For this review, take the finished solid that the model builds, in its own axes (mm). Face numbers are marked on the shaded views. A direction names the side the tool comes from. Coordinates: 2 decimals unless noted, no trailing zeros. Loops run counter-clockwise (first coordinate to the right, second up) from the corner with the lowest first, then second, coordinate; pieces in that order, holes last. Notation, with made-up numbers: (75.25, 5) -> (104.25, 5) arc R12 ccw to (104.25, 17) -> close; hole circle Ø4 at (23.25, 35). An arc over 180 degrees is marked (long way). Answer in a Markdown table with one row per item.
from build123d import *

# Parameters (mm, degrees)
RESSALTO_EXTRUS_O1_DEPTH = 10
ESBO_O3_R                = 2
CORTE_EXTRUS_O1_DEPTH    = 15
CHANFRO1_SIZE            = 1.6
FILETE1_R                = 0.5
FILETE2_R                = 0.94
RESSALTO_EXTRUS_O3_DEPTH = 10
CHANFRO5_SIZE            = 2
CHANFRO4_SIZE            = 1


with BuildPart() as part:
    # Esboço1 → Ressalto-extrusão1 (new body)
    with BuildSketch(Plane.XY):
        with BuildLine():
            Line((57, 14.25), (1.2, 14.25))
            Line((1.2, 14.25), (1.2, 4.25))
            Line((1.2, 4.25), (7.2, 4.25))
            Line((7.2, 4.25), (7.2, -0.75))
            Line((7.2, -0.75), (1.2, -0.75))
            Line((1.2, -0.75), (1.2, -15.95))
            Line((1.2, -15.95), (21.2, -15.95))
            Line((21.2, -15.95), (21.2, -20.95))
            Line((21.2, -20.95), (-3.8, -20.95))
            Line((-3.8, -20.95), (-3.8, 19.25))
            Line((-3.8, 19.25), (52, 19.25))
            Line((52, 19.25), (52, 16.25))
            Line((52, 16.25), (56.504380809, 16.25))
            ThreePointArc((56.504380809, 16.25), (56.67525574, 16.362291088), (56.829148206, 16.496918869))
            ThreePointArc((56.829148206, 16.496918869), (56.938176044, 16.51877572), (57, 16.426349589))
            Line((57, 16.426349589), (57, 16.25))
            Line((57, 16.25), (57, 14.25))
        make_face()
    extrude(amount=RESSALTO_EXTRUS_O1_DEPTH)

    # Esboço3 → Corte-extrusão1 (cut)
    with BuildSketch(Plane.XZ.offset(20.95)):
        with Locations(Location((13.2, 5, 0), (0, 0, 270))):
            Circle(ESBO_O3_R)
    extrude(amount=-CORTE_EXTRUS_O1_DEPTH, mode=Mode.SUBTRACT)

    # Chanfro1
    chanfro1_edges = [part.edges().sort_by_distance(p)[0] for p in [
        (13.2, -20.95, 7),
    ]]
    chamfer(chanfro1_edges, length=CHANFRO1_SIZE)

    # Filete1
    filete1_edges = [part.edges().sort_by_distance(p)[0] for p in [
        (13.2, -15.95, 7),
    ]]
    fillet(filete1_edges, radius=FILETE1_R)

    # Filete2
    filete2_edges = [part.edges().sort_by_distance(p)[0] for p in [
        (52, 16.25, 5),
    ]]
    fillet(filete2_edges, radius=FILETE2_R)

    # Esboço5 → Ressalto-extrusão3 (add)
    with BuildSketch(Plane.XY.offset(10)):
        Polygon((52, 19.25), (52, 21.25), (50, 21.25), (48, 19.25), align=None)
    extrude(amount=-RESSALTO_EXTRUS_O3_DEPTH)

    # Chanfro5
    chanfro5_edges = [part.edges().sort_by_distance(p)[0] for p in [
        (21.2, -20.95, 5),
        (-3.8, -20.95, 5),
        (-3.8, 19.25, 5),
        (7.2, 4.25, 5),
    ]]
    chamfer(chanfro5_edges, length=CHANFRO5_SIZE)

    # Chanfro4
    chanfro4_edges = [part.edges().sort_by_distance(p)[0] for p in [
        (1.2, 9.25, 10),
        (29.1, 14.25, 10),
        (29.1, 14.25, 0),
        (1.2, 9.25, 0),
        (7.2, 0.75, 0),
        (57, 14.25, 5),
        (7.2, 0.75, 10),
        (23.1, 19.25, 0),
        (23.1, 19.25, 10),
        (49, 20.25, 10),
        (49, 20.25, 0),
        (8.7, -20.95, 0),
        (8.7, -20.95, 10),
        (21.2, -17.45, 0),
        (-3.8, -0.85, 0),
        (3.2, 4.25, 0),
        (-2.8, 18.25, 0),
        (6.2, 3.25, 0),
        (20.2, -19.95, 0),
        (-2.8, -19.95, 0),
        (-3.8, -0.85, 10),
        (3.2, 4.25, 10),
        (21.2, -17.45, 10),
        (-2.8, 18.25, 10),
        (6.2, 3.25, 10),
        (20.2, -19.95, 10),
        (-2.8, -19.95, 10),
    ]]
    chamfer(chanfro4_edges, length=CHANFRO4_SIZE)


solid = part.part
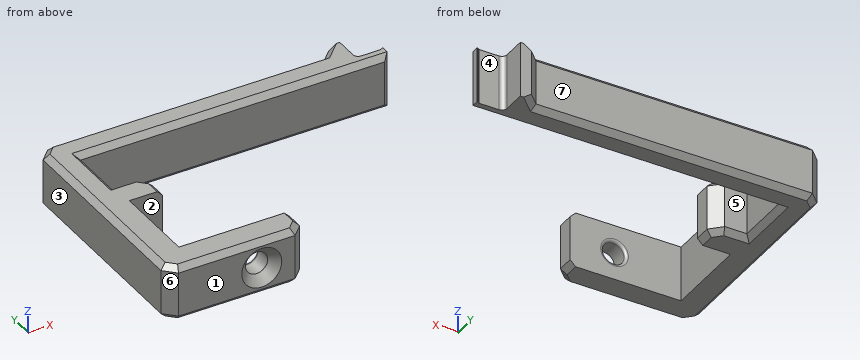
Item 1: Insertion check: pin 1 (5 mm diameter, centred on x = 14.5, z = 3.5, fed in from +Y); pin 2 (1.5 mm diameter, centred on y = -17.5, z = 3, fed in from +X); pin 3 (3 mm diameter, centred on y = -7.5, z = 4.5, fed in from +X). Each pin has a flat end and moves straight along its axis. Give the tip position at first contact, or say it passes through.
Worked answers:
| item | result |
|---|---|
| pin 1 | y = 19.25 |
| pin 2 | x = 21.2 |
| pin 3 | x = 1.2 |
Item 2: Take a section at D-D, the plane x = 44. State the section outline as (y, z) points.
Worked answers:
| item | result |
|---|---|
| outline | (14.25, 1) -> (15.25, 0) -> (18.25, 0) -> (19.25, 1) -> (19.25, 9) -> (18.25, 10) -> (15.25, 10) -> (14.25, 9) -> close |
Item 3: The part is to be moulded in two halves that separate along Y. For the marked faces 1, 2, 3 and 4, say which applies: +Y half, -Y half, draft (parallel to the pull), parting line (faces both ways), or undercut.
Worked answers:
| item | result |
|---|---|
| face 1 | -Y half |
| face 2 | undercut |
| face 3 | draft |
| face 4 | +Y half |
Item 4: For L1, parallel to Y at x = 6, z = 0.5; L2, parallel to Z at x = 13, y = -17; L3, parallel to Y at x = 9.5, z = 4, list the stretches that pass through material, from the lowest coordinate up.
Worked answers:
| item | result |
|---|---|
| L1 | -20.45 to -15.95, -0.75 to 2.74, 14.75 to 18.75 |
| L2 | 0 to 3.01, 6.99 to 10 |
| L3 | -20.95 to -15.95, 14.25 to 19.25 |
Item 5: For the marked faces 5, 6 and 7, list the 3-axis set-ups (+Z, -Z, +X, -X, +Y, -Y) from which the entire face can be reached by the end or side of a thin tool; tool diameter is ignored.
Worked answers:
| item | result |
|---|---|
| face 5 | +Z, -Z, +X |
| face 6 | +Z, -Z, -X, -Y |
| face 7 | +Z, -Z, -X, +Y |
Item 6: Take a section at C-C, the plane y = 12. State the section outline as (x, z) points.
Worked answers:
| item | result |
|---|---|
| outline | (-3.8, 1) -> (-2.8, 0) -> (0.2, 0) -> (1.2, 1) -> (1.2, 9) -> (0.2, 10) -> (-2.8, 10) -> (-3.8, 9) -> close |
Item 7: Take a section at A-A, the plane x = 13.2. State the section outline as (y, z) points, and give its area (3 significant figures).
Worked answers:
| item | result |
|---|---|
| outline | (-20.95, 1) -> (-19.95, 0) -> (-15.95, 0) -> (-15.95, 2.5) arc R0.5 ccw to (-16.45, 3) -> (-19.35, 3) -> (-20.95, 1.4) -> close; (-20.95, 8.6) -> (-19.35, 7) -> (-16.45, 7) arc R0.5 ccw to (-15.95, 7.5) -> (-15.95, 10) -> (-19.95, 10) -> (-20.95, 9) -> close; (14.25, 1) -> (15.25, 0) -> (18.25, 0) -> (19.25, 1) -> (19.25, 9) -> (18.25, 10) -> (15.25, 10) -> (14.25, 9) -> close |
| area | 74.3 mm² |
